from build123d import *

# Parameters (mm, degrees)
F1_DEPTH = 25


with BuildPart() as f1:
    # F0 (on Top) → F1 (new body)
    with BuildSketch(Plane.XY):
        Polygon((-43.5326099396, -33.3906054708), (0, 0), (-43.5326099396, 34.891307354), align=None)
        Polygon((-43.5326099396, 34.891307354), (0, 0), (45.4891324043, 34.891307354), align=None)
        with BuildLine():
            Line((-2.9963482407, 15.9782618284), (-3.8954226515, 15.9782618284))
            Line((-3.8954226515, 15.9782618284), (-4.1359542471, 17.1178678348))
            Line((-4.1359542471, 17.1178678348), (-4.1943357024, 17.1178678348))
            add(Edge.make_bspline(
                [(-4.1943357024, 17.1178678348), (-4.7921618041, 16.3659146913), (-5.3864850185, 16.0985276262)],
                knots=[0, 0, 0, 1, 1, 1], degree=2))
            add(Edge.make_bspline(
                [(-5.3864850185, 16.0985276262), (-5.9808082329, 15.8311405612), (-6.872876869, 15.8311405612)],
                knots=[0, 0, 0, 1, 1, 1], degree=2))
            add(Edge.make_bspline(
                [(-6.872876869, 15.8311405612), (-8.0615232978, 15.8311405612), (-8.7364129205, 16.4453134704)],
                knots=[0, 0, 0, 1, 1, 1], degree=2))
            add(Edge.make_bspline(
                [(-8.7364129205, 16.4453134704), (-9.4113025431, 17.0594863796), (-9.4113025431, 18.1897513531)],
                knots=[0, 0, 0, 1, 1, 1], degree=2))
            add(Edge.make_bspline(
                [(-9.4113025431, 18.1897513531), (-9.4113025431, 20.6114141167), (-5.537109173, 20.7281770272)],
                knots=[0, 0, 0, 1, 1, 1], degree=2))
            Line((-5.537109173, 20.7281770272), (-4.1803241531, 20.7725469332))
            Line((-4.1803241531, 20.7725469332), (-4.1803241531, 21.2699569319))
            add(Edge.make_bspline(
                [(-4.1803241531, 21.2699569319), (-4.1803241531, 22.2110659904), (-4.5843238234, 22.6594355667)],
                knots=[0, 0, 0, 1, 1, 1], degree=2))
            add(Edge.make_bspline(
                [(-4.5843238234, 22.6594355667), (-4.9883234937, 23.107805143), (-5.8803921299, 23.107805143)],
                knots=[0, 0, 0, 1, 1, 1], degree=2))
            add(Edge.make_bspline(
                [(-5.8803921299, 23.107805143), (-6.8798826437, 23.107805143), (-8.140922077, 22.495967492)],
                knots=[0, 0, 0, 1, 1, 1], degree=2))
            Line((-8.140922077, 22.495967492), (-8.5145633905, 23.4230650013))
            add(Edge.make_bspline(
                [(-8.5145633905, 23.4230650013), (-7.9237430635, 23.7429953761), (-7.2196627132, 23.9251455164)],
                knots=[0, 0, 0, 1, 1, 1], degree=2))
            add(Edge.make_bspline(
                [(-7.2196627132, 23.9251455164), (-6.5155823629, 24.1072956568), (-5.8056638671, 24.1072956568)],
                knots=[0, 0, 0, 1, 1, 1], degree=2))
            add(Edge.make_bspline(
                [(-5.8056638671, 24.1072956568), (-4.3764858427, 24.1072956568), (-3.6864170417, 23.4732730528)],
                knots=[0, 0, 0, 1, 1, 1], degree=2))
            add(Edge.make_bspline(
                [(-3.6864170417, 23.4732730528), (-2.9963482407, 22.8392504489), (-2.9963482407, 21.438095523)],
                knots=[0, 0, 0, 1, 1, 1], degree=2))
            Line((-2.9963482407, 21.438095523), (-2.9963482407, 15.9782618284))
        make_face(mode=Mode.SUBTRACT)
        with BuildLine():
            Line((-10.2730128225, 23.9765211971), (-10.2730128225, 23.0354121385))
            Line((-10.2730128225, 23.0354121385), (-12.3093579815, 23.0354121385))
            Line((-12.3093579815, 23.0354121385), (-12.3093579815, 15.9782618284))
            Line((-12.3093579815, 15.9782618284), (-13.5213569924, 15.9782618284))
            Line((-13.5213569924, 15.9782618284), (-13.5213569924, 23.0354121385))
            Line((-13.5213569924, 23.0354121385), (-14.9505350168, 23.0354121385))
            Line((-14.9505350168, 23.0354121385), (-14.9505350168, 23.5818625596))
            Line((-14.9505350168, 23.5818625596), (-13.5213569924, 24.020891103))
            Line((-13.5213569924, 24.020891103), (-13.5213569924, 24.4645901629))
            add(Edge.make_bspline(
                [(-13.5213569924, 24.4645901629), (-13.5213569924, 27.4140212819), (-10.945567187, 27.4140212819)],
                knots=[0, 0, 0, 1, 1, 1], degree=2))
            add(Edge.make_bspline(
                [(-10.945567187, 27.4140212819), (-10.3103769539, 27.4140212819), (-9.4556724491, 27.159478137)],
                knots=[0, 0, 0, 1, 1, 1], degree=2))
            Line((-9.4556724491, 27.159478137), (-9.7709323074, 26.1880107218))
            add(Edge.make_bspline(
                [(-9.7709323074, 26.1880107218), (-10.4715097704, 26.4145307681), (-10.9665845108, 26.4145307681)],
                knots=[0, 0, 0, 1, 1, 1], degree=2))
            add(Edge.make_bspline(
                [(-10.9665845108, 26.4145307681), (-11.6531504245, 26.4145307681), (-11.981254203, 25.9579877881)],
                knots=[0, 0, 0, 1, 1, 1], degree=2))
            add(Edge.make_bspline(
                [(-11.981254203, 25.9579877881), (-12.3093579815, 25.5014448081), (-12.3093579815, 24.4949485196)],
                knots=[0, 0, 0, 1, 1, 1], degree=2))
            Line((-12.3093579815, 24.4949485196), (-12.3093579815, 23.9765211971))
            Line((-12.3093579815, 23.9765211971), (-10.2730128225, 23.9765211971))
        make_face(mode=Mode.SUBTRACT)
        Polygon((45.4891324043, 34.891307354), (0, 0), (45.4891324043, -31.6304340959), align=None)
        with BuildLine():
            add(Edge.make_bspline(
                [(25.8402686661, 5.2373468753), (26.9161857823, 6.759086001), (29.0353264006, 6.759086001)],
                knots=[0, 0, 0, 1, 1, 1], degree=2))
            add(Edge.make_bspline(
                [(29.0353264006, 6.759086001), (31.0415254433, 6.759086001), (32.1516222469, 5.3889263585)],
                knots=[0, 0, 0, 1, 1, 1], degree=2))
            add(Edge.make_bspline(
                [(32.1516222469, 5.3889263585), (33.2617190504, 4.0187667161), (33.2617190504, 1.5132470229)],
                knots=[0, 0, 0, 1, 1, 1], degree=2))
            add(Edge.make_bspline(
                [(33.2617190504, 1.5132470229), (33.2617190504, -0.9952448171), (32.1427058067, -2.3847234133)],
                knots=[0, 0, 0, 1, 1, 1], degree=2))
            add(Edge.make_bspline(
                [(32.1427058067, -2.3847234133), (31.0236925629, -3.7742020095), (29.0353264006, -3.7742020095)],
                knots=[0, 0, 0, 1, 1, 1], degree=2))
            add(Edge.make_bspline(
                [(29.0353264006, -3.7742020095), (28.0396572462, -3.7742020095), (27.2178586754, -3.4071418883)],
                knots=[0, 0, 0, 1, 1, 1], degree=2))
            add(Edge.make_bspline(
                [(27.2178586754, -3.4071418883), (26.3960601046, -3.0400817672), (25.8402686661, -2.2762400577)],
                knots=[0, 0, 0, 1, 1, 1], degree=2))
            Line((25.8402686661, -2.2762400577), (25.7273270904, -2.2762400577))
            Line((25.7273270904, -2.2762400577), (25.4033630968, -3.5869567655))
            Line((25.4033630968, -3.5869567655), (24.2977245133, -3.5869567655))
            Line((24.2977245133, -3.5869567655), (24.2977245133, 10.8665927816))
            Line((24.2977245133, 10.8665927816), (25.8402686661, 10.8665927816))
            Line((25.8402686661, 10.8665927816), (25.8402686661, 7.3535153469))
            add(Edge.make_bspline(
                [(25.8402686661, 7.3535153469), (25.8402686661, 6.1735730952), (25.7659649978, 5.2373468753)],
                knots=[0, 0, 0, 1, 1, 1], degree=2))
            Line((25.7659649978, 5.2373468753), (25.8402686661, 5.2373468753))
        make_face(mode=Mode.SUBTRACT)
        Polygon((45.4891324043, -31.6304340959), (0, 0), (-43.5326099396, -33.3906054708), align=None)
        with BuildLine():
            ThreePointArc((45.4891324043, 34.891307354), (0.9782612324, 55.2115185664), (-43.5326099396, 34.891307354))
            Line((-43.5326099396, 34.891307354), (45.4891324043, 34.891307354))
        make_face()
        with BuildLine():
            Line((-43.5326099396, -33.3906054708), (-43.5326099396, 34.891307354))
            ThreePointArc((-43.5326099396, 34.891307354), (-74.4599689303, 0.7503509416), (-43.5326099396, -33.3906054708))
        make_face()
        with BuildLine():
            ThreePointArc((45.4891324043, -31.6304340959), (74.2935894706, 1.6304366291), (45.4891324043, 34.891307354))
            Line((45.4891324043, 34.891307354), (45.4891324043, -31.6304340959))
        make_face()
        with BuildLine():
            ThreePointArc((-43.5326099396, -33.3906054708), (1.4119301482, -54.4435900738), (45.4891324043, -31.6304340959))
            Line((45.4891324043, -31.6304340959), (-43.5326099396, -33.3906054708))
        make_face()
    extrude(amount=F1_DEPTH)


solid = f1.part
Source: CAD feature listing. Evaluate the final solid. Frame: model axes, mm. A direction names the side the tool comes from. Coordinates: 2 decimals unless noted, no trailing zeros. Loops run counter-clockwise (first coordinate to the right, second up) from the corner with the lowest first, then second, coordinate; pieces in that order, holes last. Notation, with made-up numbers: (39.25, -12) -> (72.25, -12) arc R27 cw to (72.25, 7) -> close; hole circle Ø5 at (-5, 53). An arc over 180 degrees is marked (long way). Answer in a Markdown table with one row per item. Add a question column.
Q1. Reachability of faces 5 (the face through (-1, 1, 0)), 6 (the face through (24.298, 4, 12)) from +Z, -Z, +X, -X, +Y, -Y: full face, straight path, thin tool, end or side. Return the list, or none.
Q2. Contact query for flat-ended pins moving along their axis: pin 1 Ø4 at (y, z) = (27.5, 11.5) entering from +X; pin 2 Ø8 at (x, z) = (12, 21.5) entering from +Y; pin 3 Ø1 at (x, z) = (-11, 18) entering from -Y. Output: stop coordinate, or through.
Q3. Section C-C on y = 44. Return the cut outline in (x, z).
Q4. Pull-direction query (Y, two-part tool) for faces 1 (the face through (-1, 1, 25)), 2 (the face through (-13.521, 19, 12)), 3 (the face through (-12.309, 20, 12)), 4 (the face through (74.287, 0.959, 12.325)); classes: pulls with the +Y half, pulls with the -Y half, needs draft (parallel to the pull), parting line crosses it, or undercut.
Q5. Ray query, line 1 along X through (y, z) = (21, 8); line 2 along X through (y, z) = (10.5, 5.5); line 3 along X through (y, z) = (3.5, 15). Return the intervals inside material, ascending.
Q6. Section A-A on y = 19. Give the number of separate pieces and of enclosed holes in the cut face, and give its area (3 significant figures).
Q7. Section D-D on x = -20.5. Return the cut outline in (y, z), and give its area (3 significant figures).
Computed values:
| question | item | result |
|---|---|---|
| 1 | face 5 | -Z, +X, -X, +Y, -Y |
| 1 | face 6 | +Z, -Z |
| 2 | pin 1 | stops at x = 64.34 |
| 2 | pin 2 | stops at y = 54.79 |
| 2 | pin 3 | stops at y = -53.41 |
| 3 | outline | (-33.59, 0) -> (35.55, 0) -> (35.55, 25) -> (-33.59, 25) -> close |
| 4 | face 1 | needs draft |
| 4 | face 2 | undercut |
| 4 | face 3 | undercut |
| 4 | face 4 | parting line crosses it |
| 5 | line 1 | x = -67.85 to -13.52, -12.31 to -4.18, -3 to 68.15 |
| 5 | line 2 | x = -73.05 to 24.3, 25.84 to 73.1 |
| 5 | line 3 | x = -74.35 to 24.3, 33.05 to 74.24 |
| 6 | separate pieces | 3 |
| 6 | enclosed holes | 0 |
| 6 | area | 3,280 mm^2 |
| 7 | outline | (-50.46, 0) -> (51.16, 0) -> (51.16, 25) -> (-50.46, 25) -> close |
| 7 | area | 2,540 mm^2 |
